Read the model definition and answer for the solid it produces. Units are mm, in the model's axes. A direction names the side the tool comes from. Coordinates: 2 decimals unless noted, no trailing zeros. Write each loop counter-clockwise with the first axis right and the second up, starting at its lowest first coordinate (ties: lowest second). Pieces come first, ordered by that corner, then holes. Notation, with made-up numbers: (-36.5, 16.25) -> (-10.5, 16.25) arc R11 ccw to (-10.5, 32.25) -> close; hole circle Ø1 at (2, 21.5). An arc over 180 degrees is marked (long way). Return JSON: item names as keys, results as strings.
from build123d import *

# Parameters (mm, degrees)
F0_W     = 28
F0_H     = 18
F1_DEPTH = 6
F2_R     = 0.9
F3_DEPTH = 18
F4_R     = 2.99999
F5_SIZE2 = 0.9
F5_SIZE  = 1.5588457268


# Not quite as in the source:
# - a fillet or chamfer is up to 0.001 mm smaller than in the source, because OpenCascade refuses the exact size


with BuildPart() as f1:
    # F0 (on Front) → F1 (new body)
    with BuildSketch(Plane.XZ):
        with Locations((9.4314706177, -13.323269397)):
            Rectangle(F0_W, F0_H)
    extrude(amount=F1_DEPTH)

    # F2 (on face) → F3 (cut)
    with BuildSketch(Plane(origin=(-4.5685293823, 0, 0), x_dir=(0, -1, 0), z_dir=(-1, 0, 0))):
        with Locations((3, -13.323269397)):
            Circle(F2_R)
    extrude(amount=-F3_DEPTH, mode=Mode.SUBTRACT)

    # F4 (radius 3 in the source; OpenCascade refuses exactly that, so slightly less here)
    f4_edges = [f1.edges().sort_by_distance(p)[0] for p in [
        (23.431471, -6, -13.323269),
        (23.431471, 0, -13.323269),
    ]]
    fillet(f4_edges, radius=F4_R)

    # F5
    f5_edges = [f1.edges().sort_by_distance(p)[0] for p in [
        (13.431471, -2.1, -13.323269),
    ]]
    f5_side = f1.faces().sort_by_distance((4.431471, -2.1, -13.323269))[0]
    chamfer(f5_edges, length=F5_SIZE, length2=F5_SIZE2, reference=f5_side)


solid = f1.part
1. Consider L1, parallel to Z at x = -0.75, y = -3; L2, parallel to Y at x = -1.5, z = -13.25; L3, parallel to X at y = -3.2, z = -5.5. Determine where each line is inside the solid, lowest interval first.
Taken from the geometry:
{"L1": "z = -22.32 to -14.22, -12.42 to -4.32", "L2": "y = -6 to -3.9, -2.1 to 0", "L3": "x = -4.57 to 23.42"}
2. A tool of negligible diameter and unlimited length cuts with its end or side. For faces 1 (the face through (8, 0, -13)), 2 (the face through (3.54, -3.48, -12.56)), from which of +Z, -Z, +X, -X, +Y, -Y can it reach the whole face along a straight path? Write none if from no direction.
Taken from the geometry:
{"face 1": "+Z, -Z, +X, -X, +Y", "face 2": "-X"}
3. The part is cut by section B-B (x = 1.25). Determine the outline of the cut face in (y, z), then the cut area to 3 significant figures.
Taken from the geometry:
{"outline": "(-6, -22.32) -> (0, -22.32) -> (0, -4.32) -> (-6, -4.32) -> close; hole circle Ø1.8 at (-3, -13.32)", "area": "105 mm2"}
4. Flat-ended cylindrical pins translate along their axes: pin 1 Ø2 at (y, z) = (-5, -8.5) entering from +X; pin 2 Ø1.4 at (y, z) = (-3, -13.32) entering from -X. Find the tip coordinate at first contact, or state that the pin passes through.
Taken from the geometry:
{"pin 1": "stops at x = 23.26", "pin 2": "stops at x = 12.21"}
5. For a pull along Z with two mould halves and no side action, classify faces 3 (the face through (9, -3, -22.323)), 4 (the face through (22.529, -0.855, -13.197)), 5 (the face through (9, -3, -4.323)), 6 (the face through (12.836, -2.955, -12.982)) as +Z half, -Z half, draft (parallel to the pull), parting line (faces both ways), or undercut.
Taken from the geometry:
{"face 3": "-Z half", "face 4": "draft", "face 5": "+Z half", "face 6": "undercut"}
6. The part is cut by section C-C (y = -4.85). Determine the outline of the cut face in (x, z), then the cut area to 3 significant figures.
Taken from the geometry:
{"outline": "(-4.57, -22.32) -> (22.79, -22.32) -> (22.79, -4.32) -> (-4.57, -4.32) -> close", "area": "493 mm2"}
